Verification items for the finished model (mm, model axes). A direction names the side the tool comes from. Coordinates: 2 decimals unless noted, no trailing zeros. Order: outer loops, then holes, each group sorted by start corner. A loop starts at its lowest first (then second) coordinate and runs counter-clockwise, first axis right, second up.
Q1. Draft check along X on faces 3 (the cylindrical face through (18.2, 4.83, -220.12)), 4 (the flat face through (6.35, 5, -161)), 5 (the flat face through (38.1, 5, -42)), 6 (the flat face through (3, 5, -25.4)). Enter one of: pulls with the +X half, pulls with the -X half, needs draft (parallel to the pull), parting line crosses it, or undercut.
Q2. Depth check by flat-ended pin: P1, Ø4, axis at x = 18.75, z = -101.95, coming from the +Y side. Enter the tip coordinate at first touch or a pass-through.
Q3. Cross-section at A-A, the plane x = 9.75. Record the boundary of the cut face in (y, z) (3 decimals), and give its area (3 significant figures).
Q4. Thickness scan on line 1 (Z direction, x = 28.35, y = 7.5); line 2 (Z direction, x = 6, y = 7.5); line 3 (X direction, y = 4.25, z = -204.6). Record the ranges inside material, lowest first.
Q5. Cross-section at B-B, the plane z = -92.95. Record the boundary of the cut face in (x, y) (3 decimals).
Q6. Set-up check for faces 1 (the flat face through (3, 5, -55.4)), 2 (the cylindrical face through (18.8, 4.83, -46.92)): record each of +Z, -Z, +X, -X, +Y, -Y from which the full face is reachable in a straight line by a thin tool's end or side.
Q7. Cross-section at C-C, the plane y = 4.25. Count the separate pieces of the cut face and the enclosed holes in it, and give its area (3 significant figures).
from build123d import *

# Parameters (mm, degrees)
BOSS_EXTRUDE1_DEPTH = 9.525
CUT_EXTRUDE1_REACH  = 11.525
SKETCH2_R           = 2.54
SKETCH2_W           = 6.35
SKETCH2_H           = 30


with BuildPart() as part:
    # Sketch1 → Boss-Extrude1 (new body)
    with BuildSketch(Plane(origin=(0, 0, 0), x_dir=(1, 0, 0), z_dir=(0, 1, 0))):
        with BuildLine():
            Line((6.35, 0), (31.75, 0))
            ThreePointArc((31.75, 0), (36.240128061, 1.859871939), (38.1, 6.35))
            Line((38.1, 6.35), (38.1, 247.65))
            ThreePointArc((38.1, 247.65), (36.240128061, 252.140128061), (31.75, 254))
            Line((31.75, 254), (6.35, 254))
            ThreePointArc((6.35, 254), (1.859871939, 252.140128061), (0, 247.65))
            Line((0, 247.65), (0, 6.35))
            ThreePointArc((0, 6.35), (1.859871939, 1.859871939), (6.35, 0))
        make_face()
    extrude(amount=BOSS_EXTRUDE1_DEPTH)

    # Sketch2 → Cut-Extrude1 (cut, up to next)
    with BuildSketch(Plane(origin=(0, 9.525, 0), x_dir=(1, 0, 0), z_dir=(0, 1, 0)), mode=Mode.PRIVATE) as cut_extrude1_sk1:
        with Locations((28.34999918, 40.4)):
            Circle(SKETCH2_R)
    cut_extrude1_tool1 = extrude(cut_extrude1_sk1.sketch, amount=-CUT_EXTRUDE1_REACH, mode=Mode.PRIVATE) & part.part
    add(cut_extrude1_tool1.solids().sort_by_distance((28.349999, 9.525, -40.4))[0], mode=Mode.SUBTRACT)
    # Sketch2 → Cut-Extrude1 (cut, up to next)
    with BuildSketch(Plane(origin=(0, 9.525, 0), x_dir=(1, 0, 0), z_dir=(0, 1, 0)), mode=Mode.PRIVATE) as cut_extrude1_sk2:
        with Locations((19.3499994, 49.39999978)):
            Circle(SKETCH2_R)
    cut_extrude1_tool2 = extrude(cut_extrude1_sk2.sketch, amount=-CUT_EXTRUDE1_REACH, mode=Mode.PRIVATE) & part.part
    add(cut_extrude1_tool2.solids().sort_by_distance((19.349999, 9.525, -49.4))[0], mode=Mode.SUBTRACT)
    # Sketch2 → Cut-Extrude1 (cut, up to next)
    with BuildSketch(Plane(origin=(0, 9.525, 0), x_dir=(1, 0, 0), z_dir=(0, 1, 0)), mode=Mode.PRIVATE) as cut_extrude1_sk3:
        with Locations((19.3499994, 31.40000022)):
            Circle(SKETCH2_R)
    cut_extrude1_tool3 = extrude(cut_extrude1_sk3.sketch, amount=-CUT_EXTRUDE1_REACH, mode=Mode.PRIVATE) & part.part
    add(cut_extrude1_tool3.solids().sort_by_distance((19.349999, 9.525, -31.4))[0], mode=Mode.SUBTRACT)
    # Sketch2 → Cut-Extrude1 (cut, up to next)
    with BuildSketch(Plane(origin=(0, 9.525, 0), x_dir=(1, 0, 0), z_dir=(0, 1, 0)), mode=Mode.PRIVATE) as cut_extrude1_sk4:
        with Locations((28.34999918, 161.05)):
            Circle(SKETCH2_R)
    cut_extrude1_tool4 = extrude(cut_extrude1_sk4.sketch, amount=-CUT_EXTRUDE1_REACH, mode=Mode.PRIVATE) & part.part
    add(cut_extrude1_tool4.solids().sort_by_distance((28.349999, 9.525, -161.05))[0], mode=Mode.SUBTRACT)
    # Sketch2 → Cut-Extrude1 (cut, up to next)
    with BuildSketch(Plane(origin=(0, 9.525, 0), x_dir=(1, 0, 0), z_dir=(0, 1, 0)), mode=Mode.PRIVATE) as cut_extrude1_sk5:
        with Locations((19.3499994, 170.04999978)):
            Circle(SKETCH2_R)
    cut_extrude1_tool5 = extrude(cut_extrude1_sk5.sketch, amount=-CUT_EXTRUDE1_REACH, mode=Mode.PRIVATE) & part.part
    add(cut_extrude1_tool5.solids().sort_by_distance((19.349999, 9.525, -170.05))[0], mode=Mode.SUBTRACT)
    # Sketch2 → Cut-Extrude1 (cut, up to next)
    with BuildSketch(Plane(origin=(0, 9.525, 0), x_dir=(1, 0, 0), z_dir=(0, 1, 0)), mode=Mode.PRIVATE) as cut_extrude1_sk6:
        with Locations((19.3499994, 152.05000022)):
            Circle(SKETCH2_R)
    cut_extrude1_tool6 = extrude(cut_extrude1_sk6.sketch, amount=-CUT_EXTRUDE1_REACH, mode=Mode.PRIVATE) & part.part
    add(cut_extrude1_tool6.solids().sort_by_distance((19.349999, 9.525, -152.05))[0], mode=Mode.SUBTRACT)
    # Sketch2 → Cut-Extrude1 (cut, up to next)
    with BuildSketch(Plane(origin=(0, 9.525, 0), x_dir=(1, 0, 0), z_dir=(0, 1, 0)), mode=Mode.PRIVATE) as cut_extrude1_sk7:
        with Locations((9.75000082, 213.6)):
            Circle(SKETCH2_R)
    cut_extrude1_tool7 = extrude(cut_extrude1_sk7.sketch, amount=-CUT_EXTRUDE1_REACH, mode=Mode.PRIVATE) & part.part
    add(cut_extrude1_tool7.solids().sort_by_distance((9.750001, 9.525, -213.6))[0], mode=Mode.SUBTRACT)
    # Sketch2 → Cut-Extrude1 (cut, up to next)
    with BuildSketch(Plane(origin=(0, 9.525, 0), x_dir=(1, 0, 0), z_dir=(0, 1, 0)), mode=Mode.PRIVATE) as cut_extrude1_sk8:
        with Locations((18.7500006, 222.59999978)):
            Circle(SKETCH2_R)
    cut_extrude1_tool8 = extrude(cut_extrude1_sk8.sketch, amount=-CUT_EXTRUDE1_REACH, mode=Mode.PRIVATE) & part.part
    add(cut_extrude1_tool8.solids().sort_by_distance((18.750001, 9.525, -222.6))[0], mode=Mode.SUBTRACT)
    # Sketch2 → Cut-Extrude1 (cut, up to next)
    with BuildSketch(Plane(origin=(0, 9.525, 0), x_dir=(1, 0, 0), z_dir=(0, 1, 0)), mode=Mode.PRIVATE) as cut_extrude1_sk9:
        with Locations((18.7500006, 204.60000022)):
            Circle(SKETCH2_R)
    cut_extrude1_tool9 = extrude(cut_extrude1_sk9.sketch, amount=-CUT_EXTRUDE1_REACH, mode=Mode.PRIVATE) & part.part
    add(cut_extrude1_tool9.solids().sort_by_distance((18.750001, 9.525, -204.6))[0], mode=Mode.SUBTRACT)
    # Sketch2 → Cut-Extrude1 (cut, up to next)
    with BuildSketch(Plane(origin=(0, 9.525, 0), x_dir=(1, 0, 0), z_dir=(0, 1, 0)), mode=Mode.PRIVATE) as cut_extrude1_sk10:
        with Locations((9.75000082, 92.95)):
            Circle(SKETCH2_R)
    cut_extrude1_tool10 = extrude(cut_extrude1_sk10.sketch, amount=-CUT_EXTRUDE1_REACH, mode=Mode.PRIVATE) & part.part
    add(cut_extrude1_tool10.solids().sort_by_distance((9.750001, 9.525, -92.95))[0], mode=Mode.SUBTRACT)
    # Sketch2 → Cut-Extrude1 (cut, up to next)
    with BuildSketch(Plane(origin=(0, 9.525, 0), x_dir=(1, 0, 0), z_dir=(0, 1, 0)), mode=Mode.PRIVATE) as cut_extrude1_sk11:
        with Locations((18.7500006, 101.94999978)):
            Circle(SKETCH2_R)
    cut_extrude1_tool11 = extrude(cut_extrude1_sk11.sketch, amount=-CUT_EXTRUDE1_REACH, mode=Mode.PRIVATE) & part.part
    add(cut_extrude1_tool11.solids().sort_by_distance((18.750001, 9.525, -101.95))[0], mode=Mode.SUBTRACT)
    # Sketch2 → Cut-Extrude1 (cut, up to next)
    with BuildSketch(Plane(origin=(0, 9.525, 0), x_dir=(1, 0, 0), z_dir=(0, 1, 0)), mode=Mode.PRIVATE) as cut_extrude1_sk12:
        with Locations((18.7500006, 83.95000022)):
            Circle(SKETCH2_R)
    cut_extrude1_tool12 = extrude(cut_extrude1_sk12.sketch, amount=-CUT_EXTRUDE1_REACH, mode=Mode.PRIVATE) & part.part
    add(cut_extrude1_tool12.solids().sort_by_distance((18.750001, 9.525, -83.95))[0], mode=Mode.SUBTRACT)
    # Sketch2 → Cut-Extrude1 (cut, up to next)
    with BuildSketch(Plane(origin=(0, 9.525, 0), x_dir=(1, 0, 0), z_dir=(0, 1, 0)), mode=Mode.PRIVATE) as cut_extrude1_sk13:
        with Locations((3.175, 40.4)):
            Rectangle(SKETCH2_W, SKETCH2_H)
    cut_extrude1_tool13 = extrude(cut_extrude1_sk13.sketch, amount=-CUT_EXTRUDE1_REACH, mode=Mode.PRIVATE) & part.part
    add(cut_extrude1_tool13.solids().sort_by_distance((3.175, 9.525, -40.4))[0], mode=Mode.SUBTRACT)
    # Sketch2 → Cut-Extrude1 (cut, up to next)
    with BuildSketch(Plane(origin=(0, 9.525, 0), x_dir=(1, 0, 0), z_dir=(0, 1, 0)), mode=Mode.PRIVATE) as cut_extrude1_sk14:
        with Locations((3.175, 161.05)):
            Rectangle(SKETCH2_W, SKETCH2_H)
    cut_extrude1_tool14 = extrude(cut_extrude1_sk14.sketch, amount=-CUT_EXTRUDE1_REACH, mode=Mode.PRIVATE) & part.part
    add(cut_extrude1_tool14.solids().sort_by_distance((3.175, 9.525, -161.05))[0], mode=Mode.SUBTRACT)
    # Sketch2 → Cut-Extrude1 (cut, up to next)
    with BuildSketch(Plane(origin=(0, 9.525, 0), x_dir=(1, 0, 0), z_dir=(0, 1, 0)), mode=Mode.PRIVATE) as cut_extrude1_sk15:
        with Locations((34.925, 213.6)):
            Rectangle(SKETCH2_W, SKETCH2_H)
    cut_extrude1_tool15 = extrude(cut_extrude1_sk15.sketch, amount=-CUT_EXTRUDE1_REACH, mode=Mode.PRIVATE) & part.part
    add(cut_extrude1_tool15.solids().sort_by_distance((34.925, 9.525, -213.6))[0], mode=Mode.SUBTRACT)
    # Sketch2 → Cut-Extrude1 (cut, up to next)
    with BuildSketch(Plane(origin=(0, 9.525, 0), x_dir=(1, 0, 0), z_dir=(0, 1, 0)), mode=Mode.PRIVATE) as cut_extrude1_sk16:
        with Locations((34.925, 92.95)):
            Rectangle(SKETCH2_W, SKETCH2_H)
    cut_extrude1_tool16 = extrude(cut_extrude1_sk16.sketch, amount=-CUT_EXTRUDE1_REACH, mode=Mode.PRIVATE) & part.part
    add(cut_extrude1_tool16.solids().sort_by_distance((34.925, 9.525, -92.95))[0], mode=Mode.SUBTRACT)


solid = part.part
Check values:
1. face 3: undercut
1. face 4: pulls with the -X half
1. face 5: pulls with the +X half
1. face 6: needs draft
2. P1: passes through
3. outline: (0, -254) - (9.525, -254) - (9.525, -216.14) - (0, -216.14) - close; (0, -211.06) - (9.525, -211.06) - (9.525, -95.49) - (0, -95.49) - close; (0, -90.41) - (9.525, -90.41) - (9.525, 0) - (0, 0) - close
3. area: 2,320 mm2
4. line 1: z = -254 to -163.59, -158.51 to -42.94, -37.86 to 0
4. line 2: z = -253.99 to -176.05, -146.05 to -55.4, -25.4 to -0.01
4. line 3: x = 0 to 16.21, 21.29 to 31.75
5. outline: (0, 0) - (7.21, 0) - (7.21, 9.525) - (0, 9.525) - close; (12.29, 0) - (31.75, 0) - (31.75, 9.525) - (12.29, 9.525) - close
6. face 1: -X, +Y, -Y
6. face 2: +Y, -Y
7. separate pieces: 1
7. enclosed holes: 12
7. area: 8,640 mm2
